Here's how the part is built. I have some questions about the finished solid (model axes, mm). A direction names the side the tool comes from. Coordinates: 2 decimals unless noted, no trailing zeros. Loops run counter-clockwise (first coordinate to the right, second up) from the corner with the lowest first, then second, coordinate; pieces in that order, holes last. Notation, with made-up numbers: (-34.75, 85.5) -> (18.25, 85.5) arc R26 ccw to (18.25, 118.5) -> close; hole circle Ø1 at (42.5, 76.5). An arc over 180 degrees is marked (long way). Answer as a JSON object with one key per item and string values. Group by question number.
Q1. I want a section at C-C on x = 6. Write out the boundary of the cut face in (y, z) (3 decimals).
Q2. I need wall thicknesses on line 1 (X direction, y = -1.5, z = -1.3) (3 decimals); line 2 (Y direction, x = 15.15, z = 0.2) (3 decimals); line 3 (Y direction, x = 7.8, z = -1.5). Which ranges of each line are inside material? Lowest first, please.
Q3. I want a section at B-B on x = 15.15. Write out the boundary of the cut face in (y, z) (3 decimals), then the cut area to 3 significant figures.
Q4. I want a section at A-A on y = 0. Write out the boundary of the cut face in (x, z) (3 decimals), then the cut area to 3 significant figures.
Q5. I'm going to push flat-ended pins straight in: pin 1 (4 mm diameter, centred on x = -5, y = 2, fed in from -Z); pin 2 (1.9 mm diameter, centred on x = -14.59, y = 0, fed in from -Z); pin 3 (1.5 mm diameter, centred on x = -7.5, z = -2.5, fed in from -Y); pin 4 (0.8 mm diameter, centred on y = 1, z = -1.5, fed in from -X) (3 decimals). Where does each tip first touch, or does it pass through?
Q6. Thinking about a two-plate mould opening in Y: for faces 4 (the flat face through (-10.145, -0.2, -0.2)), 5 (the flat face through (7.686, 1.788, -1.129)), 6 (the cylindrical face through (16.26, -0.46, 0.22)), which applies, released by +Y, released by -Y, zero draft, split by the parting line, or undercut?
Q7. I want a section at D-D on z = -1.4. Write out the boundary of the cut face in (x, y) (3 decimals).
Q8. On a 3-axis mill with a long thin cutter (end or side, diameter ignored), from which of +Z, -Z, +X, -X, +Y, -Y can I reach the whole of each face in a straight line? I mean faces 1 (the flat face through (10.145, -0.2, -0.2)), 2 (the cylindrical face through (7.69, 1.04, -1.36)), 3 (the flat face through (-5.295, -0.2, -0.2)). Say none if no direction works.
```python
from build123d import *

# Parameters (mm, degrees)
SKETCH1_W           = 37
SKETCH1_H           = 7.63
SKETCH1_R           = 1.2
BOSS_EXTRUDE1_DEPTH = 0.44
SKETCH3_R           = 1.05
BOSS_EXTRUDE2_DEPTH = 4.85


with BuildPart() as part:
    # Sketch1 → Boss-Extrude1 (new body)
    with BuildSketch(Plane.XY):
        Rectangle(SKETCH1_W, SKETCH1_H)
        with Locations((-14.59410802, 0)):
            Circle(SKETCH1_R, mode=Mode.SUBTRACT)
        with Locations((15.15, 0)):
            Circle(SKETCH1_R, mode=Mode.SUBTRACT)
    extrude(amount=BOSS_EXTRUDE1_DEPTH)

    # Sketch3 → Boss-Extrude2 (add)
    with BuildSketch(Plane(origin=(-5.295, 0, 0), x_dir=(0, 0, -1), z_dir=(1, 0, 0))):
        with BuildLine():
            Line((2.227470567, 0.890666365), (0, 2.71))
            Line((0, 2.71), (0, -2.71))
            Line((0, -2.71), (2.227470567, -0.890666365))
            ThreePointArc((2.227470567, -0.890666365), (2.65, 0), (2.227470567, 0.890666365))
        make_face()
        with Locations((1.5, 0)):
            Circle(SKETCH3_R, mode=Mode.SUBTRACT)
    boss_extrude2 = extrude(amount=-BOSS_EXTRUDE2_DEPTH)

    # Mirror1: Boss-Extrude2 across plane
    add(boss_extrude2.mirror(Plane(origin=(0, 0, 0), x_dir=(0, 0, 1), z_dir=(1, 0, 0))))


solid = part.part
```
Result set:
{
 "1": {"outline": "(-3.815, 0) -> (-2.71, 0) -> (-0.891, -2.227) arc R1.15 ccw to (0.891, -2.227) -> (2.71, 0) -> (3.815, 0) -> (3.815, 0.44) -> (-3.815, 0.44) -> close; hole circle Ø2.1 at (0, -1.5)"},
 "2": {"line 1": "x = -10.145 to -5.295, 5.295 to 10.145", "line 2": "y = -3.815 to -1.2, 1.2 to 3.815", "line 3": "y = -1.48 to -1.05, 1.05 to 1.48"},
 "3": {"outline": "(-3.815, 0) -> (-1.2, 0) -> (-1.2, 0.44) -> (-3.815, 0.44) -> close; (1.2, 0) -> (3.815, 0) -> (3.815, 0.44) -> (1.2, 0.44) -> close", "area": "2.30 mm²"},
 "4": {"outline": "(-18.5, 0) -> (-15.794, 0) -> (-15.794, 0.44) -> (-18.5, 0.44) -> close; (-13.394, 0) -> (-10.145, 0) -> (-10.145, -0.45) -> (-5.295, -0.45) -> (-5.295, 0) -> (5.295, 0) -> (5.295, -0.45) -> (10.145, -0.45) -> (10.145, 0) -> (13.95, 0) -> (13.95, 0.44) -> (-13.394, 0.44) -> close; (-10.145, -2.65) -> (-5.295, -2.65) -> (-5.295, -2.55) -> (-10.145, -2.55) -> close; (5.295, -2.65) -> (10.145, -2.65) -> (10.145, -2.55) -> (5.295, -2.55) -> close; (16.35, 0) -> (18.5, 0) -> (18.5, 0.44) -> (16.35, 0.44) -> close", "area": "19.5 mm²"},
 "5": {"pin 1": "stops at z = -2.65", "pin 2": "passes through", "pin 3": "stops at y = -1.28", "pin 4": "stops at x = -10.145"},
 "6": {"face 4": "zero draft", "face 5": "released by +Y", "face 6": "undercut"},
 "7": {"outline": "(-10.145, -1.567) -> (-5.295, -1.567) -> (-5.295, -1.045) -> (-10.145, -1.045) -> close; (-10.145, 1.045) -> (-5.295, 1.045) -> (-5.295, 1.567) -> (-10.145, 1.567) -> close; (5.295, -1.567) -> (10.145, -1.567) -> (10.145, -1.045) -> (5.295, -1.045) -> close; (5.295, 1.045) -> (10.145, 1.045) -> (10.145, 1.567) -> (5.295, 1.567) -> close"},
 "8": {"face 1": "-Z, +X, +Y, -Y", "face 2": "+X, -X", "face 3": "-Z, +Y, -Y"}
}
